Check sheet for the modelled part. Datum: model origin and axes. Units: mm. A direction names the side the tool comes from. Round coordinates to 2 decimals unless told otherwise and drop trailing zeros. Order: outer loops, then holes, each group sorted by start corner. A loop starts at its lowest first (then second) coordinate and runs counter-clockwise, first axis right, second up. Notation, with made-up numbers: (52, 37.5) -> (110, 37.5) arc R20 cw to (110, 54.5) -> close; hole circle Ø8 at (46, 59.25). An arc over 180 degrees is marked (long way). Answer in a Markdown table with one row per item. Add a question column.
1. Material ranges on L1, parallel to Y at x = -117.5, z = 19; L2, parallel to Z at x = -40, y = 32; L3, parallel to Y at x = -47.5, z = 10, recorded low to high. Write a range as from..to.
2. Depth check by flat-ended pin: P1, Ø8, axis at x = -59, y = 111, coming from the +Z side. Enter the tip coordinate at first touch or a pass-through.
3. Sectioned sample at B-B, the plane z = 11. Count the separate pieces of the cut face and the enclosed holes in it, then the cut area to 3 significant figures.
4. Access from +Z, -Z, +X, -X, +Y, -Y to the whole of each face (thin tool, end or side, straight path). Record for faces 4 (the flat face through (-9, -75, 38.1)), 5 (the flat face through (-136, 13.002, 21)), 6 (the flat face through (-96.579, -77, 22)).
5. Sectioned sample at D-D, the plane y = 99.5. Record the boundary of the cut face in (x, z).
6. Draft check along X on faces 1 (the flat face through (-74, 140.002, 21)), 2 (the flat face through (-150.554, -77, 22)), 3 (the flat face through (-161.667, -39, 19)). Enter one of: +X half, -X half, draft (parallel to the pull), parting line (faces both ways), or undercut.
7. Sectioned sample at A-A, the plane x = -5.5. Record the boundary of the cut face in (y, z) (3 decimals).
```python
from build123d import *

# Parameters (mm, degrees)
F0_W     = 177.8
F0_H     = 330.2
F1_DEPTH = 38.1
F2_W     = 177.8
F2_H     = 127
F3_DEPTH = 31.75
F4_W     = 3.175
F4_H     = 177.8
F5_DEPTH = 31.75
F6_R     = 3.175


with BuildPart() as f1:
    # F0 (on Top) → F1 (new body)
    with BuildSketch(Plane.XY):
        with Locations((-72.766965, 0.301726)):
            Rectangle(F0_W, F0_H)
    extrude(amount=F1_DEPTH)

    # F2 (on face) → F3 (cut)
    with BuildSketch(Plane.XY.offset(38.1)):
        with Locations((-72.766965, 76.501726)):
            Rectangle(F2_W, F2_H)
    extrude(amount=-F3_DEPTH, mode=Mode.SUBTRACT)

    # F4 (on face) → F5 (cut)
    with BuildSketch(Plane.XY.offset(38.1)):
        with Locations((-148.966965, -75.898274)):
            Rectangle(F4_W, F4_H)
        with Locations((-123.566965, -75.898274)):
            Rectangle(F4_W, F4_H)
        with Locations((-98.166965, -75.898274)):
            Rectangle(F4_W, F4_H)
        with Locations((-72.766965, -75.898274)):
            Rectangle(F4_W, F4_H)
        with Locations((-47.366965, -75.898274)):
            Rectangle(F4_W, F4_H)
        with Locations((-21.966965, -75.898274)):
            Rectangle(F4_W, F4_H)
        with Locations((3.433035, -75.898274)):
            Rectangle(F4_W, F4_H)
    extrude(amount=-F5_DEPTH, mode=Mode.SUBTRACT)

    # F6
    f6_edges = [f1.edges().sort_by_distance(p)[0] for p in [
        (-72.766965, 140.001726, 38.1),
        (10.576785, -164.798274, 38.1),
        (-9.266965, -164.798274, 38.1),
        (-34.666965, -164.798274, 38.1),
        (-60.066965, -164.798274, 38.1),
        (-85.466965, -164.798274, 38.1),
        (-110.866965, -164.798274, 38.1),
        (-136.266965, -164.798274, 38.1),
        (-156.110715, -164.798274, 38.1),
        (10.576785, 13.001726, 38.1),
        (-156.110715, 13.001726, 38.1),
        (-136.266965, 13.001726, 38.1),
        (-110.866965, 13.001726, 38.1),
        (-85.466965, 13.001726, 38.1),
        (-60.066965, 13.001726, 38.1),
        (-34.666965, 13.001726, 38.1),
        (-9.266965, 13.001726, 38.1),
        (-72.766965, 165.401726, 38.1),
    ]]
    fillet(f6_edges, radius=F6_R)


solid = f1.part
```
Answer key:
| question | item | result |
|---|---|---|
| 1 | L1 | y = -164.8..13, 140..165.4 |
| 1 | L2 | z = 0..6.35 |
| 1 | L3 | y = 140..165.4 |
| 2 | P1 | stops at z = 6.35 |
| 3 | separate pieces | 9 |
| 3 | enclosed holes | 0 |
| 3 | area | 32,200 mm² |
| 4 | face 4 | +Z, +X, -X, +Y, -Y |
| 4 | face 5 | +Z, +X, -X |
| 4 | face 6 | +Z, -Y |
| 5 | outline | (-161.67, 0) -> (16.13, 0) -> (16.13, 6.35) -> (-161.67, 6.35) -> close |
| 6 | face 1 | draft |
| 6 | face 2 | undercut |
| 6 | face 3 | -X half |
| 7 | outline | (-164.798, 0) -> (165.402, 0) -> (165.402, 34.925) arc R3.175 ccw to (162.227, 38.1) -> (143.177, 38.1) arc R3.175 ccw to (140.002, 34.925) -> (140.002, 6.35) -> (13.002, 6.35) -> (13.002, 34.925) arc R3.175 ccw to (9.827, 38.1) -> (-161.623, 38.1) arc R3.175 ccw to (-164.798, 34.925) -> close |
